The model under review builds one solid part; all positions refer to its coordinate system, in mm. A direction names the side the tool comes from. Give positions to 0.01 mm unless a question says otherwise; leave off trailing zeros. Loops run counter-clockwise (first coordinate to the right, second up) from the corner with the lowest first, then second, coordinate; pieces in that order, holes last. Notation, with made-up numbers: M 52,-6 L 102,-6 A23 cw 102,22 Z; hole C -35.5,-28 d10. An arc over 180 degrees is marked long. Return JSON: item names as keys, results as strings.
```python
from build123d import *

# Parameters (mm, degrees)
BOSS_EXTRUDE1_DEPTH     = 12
BOSS_EXTRUDE2_DEPTH     = 10.5
CUT_EXTRUDE1_DEPTH      = 18.839562775
CUT_EXTRUDE1_DEPTH_BACK = 18.839562775
SKETCH2_R               = 0.5
SKETCH5_R               = 1.65
CUT_EXTRUDE2_DEPTH      = 1.6
CUT_EXTRUDE5_DEPTH      = 17.947271167
CUT_EXTRUDE5_DEPTH_BACK = 17.947271167
SKETCH7_R               = 0.65


with BuildPart() as part:
    # Sketch1 → Boss-Extrude1 (new body)
    with BuildSketch(Plane(origin=(0, 0, 0), x_dir=(1, 0, 0), z_dir=(0, 1, 0))):
        Polygon((0, 0), (8, 0), (8, 2), (6, 2), (6, 7), (-6, 7), (-6, 2), (-8, 2), (-8, 0), align=None)
    extrude(amount=BOSS_EXTRUDE1_DEPTH)

    # Sketch4 → Boss-Extrude2 (add)
    with BuildSketch(Plane.XY):
        with BuildLine():
            Line((-6, 11), (-6, 1))
            ThreePointArc((-6, 1), (-5.853553391, 0.646446609), (-5.5, 0.5))
            Line((-5.5, 0.5), (5.5, 0.5))
            ThreePointArc((5.5, 0.5), (5.853553391, 0.646446609), (6, 1))
            Line((6, 1), (6, 11))
            ThreePointArc((6, 11), (5.853553391, 11.353553391), (5.5, 11.5))
            Line((5.5, 11.5), (-5.5, 11.5))
            ThreePointArc((-5.5, 11.5), (-5.853553391, 11.353553391), (-6, 11))
        make_face()
    extrude(amount=-BOSS_EXTRUDE2_DEPTH)

    # Sketch2 → Cut-Extrude1 (cut, two sides: drawn at the far end of the back side and taken through both)
    with BuildSketch(Plane(origin=(0, 12, 0), x_dir=(1, 0, 0), z_dir=(0, 1, 0)).offset(-CUT_EXTRUDE1_DEPTH_BACK)):
        with Locations(Location((-4, 5, 0), (0, 0, 270))):
            Circle(SKETCH2_R)
        with Locations(Location((4, 5, 0), (0, 0, 270))):
            Circle(SKETCH2_R)
    extrude(amount=CUT_EXTRUDE1_DEPTH + CUT_EXTRUDE1_DEPTH_BACK, mode=Mode.SUBTRACT)

    # Sketch5 → Cut-Extrude2 (cut)
    with BuildSketch(Plane(origin=(0, 0, -10.5), x_dir=(-1, 0, 0), z_dir=(0, 0, -1))):
        with Locations((3.55, 6)):
            Circle(SKETCH5_R)
        with Locations((-3.55, 6)):
            Circle(SKETCH5_R)
        with Locations((0, 6)):
            Circle(SKETCH5_R)
        with Locations((-3.55, 10.75)):
            Circle(SKETCH5_R)
        with Locations((0, 10.75)):
            Circle(SKETCH5_R)
        with Locations((3.55, 10.75)):
            Circle(SKETCH5_R)
        with Locations((-3.55, 1.25)):
            Circle(SKETCH5_R)
        with Locations((0, 1.25)):
            Circle(SKETCH5_R)
        with Locations((3.55, 1.25)):
            Circle(SKETCH5_R)
    extrude(amount=-CUT_EXTRUDE2_DEPTH, mode=Mode.SUBTRACT)

    # Sketch7 → Cut-Extrude5 (cut, two sides: drawn at the far end of the back side and taken through both)
    with BuildSketch(Plane(origin=(0, 0, -8.9), x_dir=(-1, 0, 0), z_dir=(0, 0, -1)).offset(-CUT_EXTRUDE5_DEPTH_BACK)):
        with Locations((-3.55, 6)):
            Circle(SKETCH7_R)
        with Locations((3.55, 6)):
            Circle(SKETCH7_R)
        with Locations((0, 6)):
            Circle(SKETCH7_R)
        with Locations((-3.55, 1.25)):
            Circle(SKETCH7_R)
        with Locations((0, 1.25)):
            Circle(SKETCH7_R)
        with Locations((3.55, 1.25)):
            Circle(SKETCH7_R)
        with Locations((3.55, 10.75)):
            Circle(SKETCH7_R)
        with Locations((0, 10.75)):
            Circle(SKETCH7_R)
        with Locations((-3.55, 10.75)):
            Circle(SKETCH7_R)
    extrude(amount=CUT_EXTRUDE5_DEPTH + CUT_EXTRUDE5_DEPTH_BACK, mode=Mode.SUBTRACT)


solid = part.part
```
1) Wall thickness on L1, parallel to X at y = 1.25, z = -9.7; L2, parallel to Y at x = -3.55, z = -4.5; L3, parallel to Z at x = 4, y = 9.25: over which ranges is each line inside the solid? List them lowest first. Write a range as from..to.
From the geometry:
{"L1": "-6..-5.2, -1.9..-1.65, 1.65..1.9, 5.2..6", "L2": "0..0.6, 1.9..5.35, 6.65..10.1, 11.4..12", "L3": "-8.9..-5.5, -4.5..0"}
2) Tool access review of faces 4 (the face through (-7, 6, -2)), 5 (the face through (7, 6, -2)), 6 (the face through (-2.24, 5, -9.71)): name each direction out of +Z, -Z, +X, -X, +Y, -Y from which nothing blocks a thin tool from reaching the whole face with its end or side.
From the geometry:
{"face 4": "-Z, -X, +Y, -Y", "face 5": "-Z, +X, +Y, -Y", "face 6": "-Z"}
3) Consider section A-A on x = 0. Write out the cut boundary in (y, z), then the cut area to 3 significant figures.
From the geometry:
{"outline": "M 0,-7 L 0.5,-7 L 0.5,-8.9 L 0.6,-8.9 L 0.6,0 L 0,0 Z; M 1.9,-8.9 L 2.9,-8.9 L 2.9,-10.5 L 4.35,-10.5 L 4.35,-8.9 L 5.35,-8.9 L 5.35,0 L 1.9,0 Z; M 6.65,-8.9 L 7.65,-8.9 L 7.65,-10.5 L 9.1,-10.5 L 9.1,-8.9 L 10.1,-8.9 L 10.1,0 L 6.65,0 Z; M 11.4,-8.9 L 11.5,-8.9 L 11.5,-7 L 12,-7 L 12,0 L 11.4,0 Z", "area": "74.8 mm²"}
4) The part is to be moulded in two halves that separate along X. For faces 1 (the face through (0.1, 11.8, -7)), 2 (the face through (0.39, 10.05, -8.9)), 3 (the face through (-8, 6, -1)), say which applies: released by +X, released by -X, zero draft, split by the parting line, or undercut.
From the geometry:
{"face 1": "zero draft", "face 2": "undercut", "face 3": "released by -X"}
5) Consider section D-D on y = 1.25. Count the separate pieces of the cut face and the enclosed holes in it, then the cut area to 3 significant figures.
From the geometry:
{"separate pieces": "4", "enclosed holes": "0", "area": "83.1 mm²"}
6) Insertion check: pin 1 (5.5 mm diameter, centred on x = -3.55, y = 6, fed in from +Z); pin 2 (0.7 mm diameter, centred on x = -3, y = 10, fed in from -Z); pin 3 (1.6 mm diameter, centred on x = -7, y = 8, fed in from -Z); pin 4 (1 mm diameter, centred on y = 2, z = -4, fed in from -X). Each pin has a flat end and moves straight along its axis. Give the tip position at first contact, or say it passes through.
From the geometry:
{"pin 1": "z = 0", "pin 2": "z = -8.9", "pin 3": "z = -2", "pin 4": "x = -6"}
7) Consider section B-B on y = 3.75. Write out the cut boundary in (x, z).
From the geometry:
{"outline": "M -8,-2 L -6,-2 L -6,-10.5 L 6,-10.5 L 6,-2 L 8,-2 L 8,0 L -8,0 Z; hole C -4,-5 d1; hole C 4,-5 d1"}
8) Consider section C-C on z = -5. Write out the cut boundary in (x, y), then the cut area to 3 significant figures.
From the geometry:
{"outline": "M -6,0 L -4.5,0 L -4.5,12 L -6,12 Z; M -3.5,0 L 3.5,0 L 3.5,0.6 A0.65 cw 3.5,1.9 L 3.5,5.35 A0.65 cw 3.5,6.65 L 3.5,10.1 A0.65 cw 3.5,11.4 L 3.5,12 L -3.5,12 L -3.5,11.4 A0.65 cw -3.5,10.1 L -3.5,6.65 A0.65 cw -3.5,5.35 L -3.5,1.9 A0.65 cw -3.5,0.6 Z; M 4.5,0 L 6,0 L 6,12 L 4.5,12 Z; hole C 0,1.25 d1.3; hole C 0,6 d1.3; hole C 0,10.75 d1.3", "area": "112 mm²"}
